Part model, mm, in its own coordinate system. A direction names the side the tool comes from. Round coordinates to 2 decimals unless told otherwise and drop trailing zeros. Write each loop counter-clockwise with the first axis right and the second up, starting at its lowest first coordinate (ties: lowest second). Pieces come first, ordered by that corner, then holes. Notation, with made-up numbers: M 45.25,-5 L 81.25,-5 A23 ccw 81.25,9 Z; hole C 50,-15.5 d10. An arc over 180 degrees is marked long. Use one line per item in the form item = value. Start each with the question number.
Item 1: Cut at B-B, the plane z = 4. Give the cut face in (x, y), then the cut area to 3 significant figures.
Item 2: Cut at D-D, the plane x = 1.5. Give the cut face in (y, z).
Item 3: Probe L1, parallel to Z at x = 45, y = 4.5; L2, parallel to X at y = -13, z = 16.5; L3, parallel to X at y = 0, z = 4. List the from-to ranges inside material, lowest first.
Item 4: Flat gauge pins, fed straight in: pin 1 Ø12 at (x, y) = (-45, -6) entering from +Z; pin 2 Ø4.5 at (x, z) = (40.5, 1.5) entering from +Y; pin 3 Ø6 at (y, z) = (-2.5, 31) entering from -X; pin 4 Ø12 at (x, z) = (35.5, 7) entering from -Y. Where does each tip first touch, or does it go through?
Item 5: Which spindle directions (+Z, -Z, +X, -X, +Y, -Y) get a long thin tool onto all of the face, cutting with end or side? Do faces 1 (the face through (-44, -14, 0)), 2 (the face through (-30, 7, 41)), 3 (the face through (-40, 0, -5)). Say none if no direction does.
Item 6: Cut at C-C, the plane x = -45. Give the cut face in (y, z).
Item 7: Cut at A-A, the plane y = 8.5. Give the cut face in (x, z), then the cut area to 3 significant figures.
Item 8: Mould opens along X. For faces 4 (the face through (44, -14, 0)), 5 (the face through (0, 39, 41)) say: +X half, -X half, draft (parallel to the pull), parting line (faces both ways), or undercut.
from build123d import *

# Parameters (mm, degrees)
SKETCH_1_W            = 100
SKETCH_1_H            = 28
EXTRUDE_1_DEPTH       = 20
SKETCH_2_W            = 80
SKETCH_2_H            = 10
CUT_EXTRUDE_1_DEPTH   = 59.172158289
SKETCH_3_W            = 70
SKETCH_3_H            = 10
EXTRUDE_2_DEPTH       = 25
SKETCH_4_W            = 70
SKETCH_4_H            = 10
EXTRUDE_3_DEPTH       = 12
HOLE_WIZARD_3_0_3_1_D = 3
HOLE_WIZARD_3_0_3_2_D = 3
SKETCH_13_W           = 70
SKETCH_13_H           = 5
EXTRUDE_4_DEPTH       = 10
CUT_EXTRUDE_3_DEPTH   = 10
EXTRUDE_5_DEPTH       = 74
SKETCH_17_W           = 70
SKETCH_17_H           = 5
EXTRUDE_6_DEPTH       = 70
SKETCH_18_W           = 70
SKETCH_18_H           = 89
EXTRUDE_7_DEPTH       = 8


with BuildPart() as part:
    # 草图1 → 凸台-拉伸1 (new body)
    with BuildSketch(Plane(origin=(0, 0, -10), x_dir=(-1, 0, 0), z_dir=(0, 0, -1))):
        Rectangle(SKETCH_1_W, SKETCH_1_H)
    extrude(amount=-EXTRUDE_1_DEPTH)

    # 草图2 → 切除-拉伸1 (cut, through all)
    with BuildSketch(Plane(origin=(0, 14, 0), x_dir=(-1, 0, 0), z_dir=(0, 1, 0))):
        with Locations((0, -5)):
            Rectangle(SKETCH_2_W, SKETCH_2_H)
    extrude(amount=-CUT_EXTRUDE_1_DEPTH, mode=Mode.SUBTRACT)

    # 草图3 → 凸台-拉伸2 (add)
    with BuildSketch(Plane(origin=(0, 14, 0), x_dir=(-1, 0, 0), z_dir=(0, 1, 0))):
        with Locations((0, 5)):
            Rectangle(SKETCH_3_W, SKETCH_3_H)
    extrude(amount=EXTRUDE_2_DEPTH)

    # 草图4 → 凸台-拉伸3 (add)
    with BuildSketch(Plane.XZ.offset(14)):
        with Locations((0, 5)):
            Rectangle(SKETCH_4_W, SKETCH_4_H)
    extrude(amount=EXTRUDE_3_DEPTH)

    # Ø3.0 (3) 直径孔1 (through all)
    with Locations(Plane(origin=(0, 14, 0), x_dir=(1, 0, 0), z_dir=(0, 1, 0))):
        with Locations((-45, -4), (-45, 4)):
            Hole(HOLE_WIZARD_3_0_3_1_D / 2)

    # Ø3.0 (3) 直径孔2 (through all)
    with Locations(Plane(origin=(0, -14, 0), x_dir=(-1, 0, 0), z_dir=(0, -1, 0))):
        with Locations((-45, 4), (-45, -4)):
            Hole(HOLE_WIZARD_3_0_3_2_D / 2)

    # 草图13 → 凸台-拉伸4 (add)
    with BuildSketch(Plane(origin=(0, 0, 0), x_dir=(-1, 0, 0), z_dir=(0, 0, -1))):
        with Locations((0, 41.5)):
            Rectangle(SKETCH_13_W, SKETCH_13_H)
    extrude(amount=-EXTRUDE_4_DEPTH)

    # 草图15 → 切除-拉伸3 (cut)
    with BuildSketch(Plane(origin=(0, 0, 0), x_dir=(-1, 0, 0), z_dir=(0, 0, -1))):
        Polygon((0, -26), (30, -26), (30, 39), (-30, 39), (-30, -26), align=None)
    extrude(amount=-CUT_EXTRUDE_3_DEPTH, mode=Mode.SUBTRACT)

    # 草图16 → 凸台-拉伸5 (add)
    with BuildSketch(Plane.XY.offset(10)):
        Polygon((-35, -26), (-35, 44), (35, 44), (35, -26), (30, -26), (30, 39), (-30, 39), (-30, -26), align=None)
    extrude(amount=EXTRUDE_5_DEPTH)

    # 草图17 → 凸台-拉伸6 (add)
    with BuildSketch(Plane(origin=(0, 44, 0), x_dir=(1, 0, 0), z_dir=(0, 1, 0))):
        with Locations((0, -86.5)):
            Rectangle(SKETCH_17_W, SKETCH_17_H)
    extrude(amount=-EXTRUDE_6_DEPTH)

    # 草图18 → 凸台-拉伸7 (add)
    with BuildSketch(Plane(origin=(0, 44, 0), x_dir=(1, 0, 0), z_dir=(0, 1, 0))):
        with Locations((0, -44.5)):
            Rectangle(SKETCH_18_W, SKETCH_18_H)
    extrude(amount=EXTRUDE_7_DEPTH)


solid = part.part
Model answer:
q1.outline = M -50,-14 L -46.5,-14 L -46.5,14 L -50,14 Z; M -43.5,-14 L -35,-14 L -35,-26 L -30,-26 L -30,39 L 30,39 L 30,-26 L 35,-26 L 35,-14 L 43.5,-14 L 43.5,14 L 35,14 L 35,52 L -35,52 L -35,14 L -43.5,14 Z; M 46.5,-14 L 50,-14 L 50,14 L 46.5,14 Z
q1.area = 2,230 mm²
q2.outline = M -26,84 L 39,84 L 39,0 L 52,0 L 52,89 L -26,89 Z
q3.L1 = -10 to -5.5, -2.5 to 2.5, 5.5 to 10
q3.L2 = -35 to -30, 30 to 35
q3.L3 = -50 to -46.5, -43.5 to -30, 30 to 43.5, 46.5 to 50
q4.pin_1 = 10
q4.pin_2 = 14
q4.pin_3 = -35
q4.pin_4 = -26
q5.face_1 = +Z, -Z, -X, -Y
q5.face_2 = -Z, -Y
q5.face_3 = -Z, +Y, -Y
q6.outline = M -14,-10 L 14,-10 L 14,-5.5 L -14,-5.5 Z; M -14,-2.5 L 14,-2.5 L 14,2.5 L -14,2.5 Z; M -14,5.5 L 14,5.5 L 14,10 L -14,10 Z
q7.outline = M -50,-10 L -40,-10 L -40,0 L -30,0 L -30,84 L 30,84 L 30,0 L 40,0 L 40,-10 L 50,-10 L 50,10 L 35,10 L 35,89 L -35,89 L -35,10 L -50,10 Z; hole C -45,-4 d3; hole C -45,4 d3; hole C 45,-4 d3; hole C 45,4 d3
q7.area = 1,660 mm²
q8.face_4 = draft
q8.face_5 = undercut
